Geometry check sheet. Reference: the model listing, model coordinates, mm. A direction names the side the tool comes from. Give positions to 0.01 mm unless a question says otherwise; leave off trailing zeros. Write each loop counter-clockwise with the first axis right and the second up, starting at its lowest first coordinate (ties: lowest second). Pieces come first, ordered by that corner, then holes. Notation, with made-up numbers: M 26,-35.5 L 71,-35.5 A26 cw 71,-21.5 Z; hole C 71.25,86 d11. An arc over 180 degrees is marked long. One line per item, written item: value. Start each with the question number.
1. Gauge pin test, flat ends, axial feed: pin 1 (3 mm diameter, centred on x = 10, z = 57, fed in from +Y); pin 2 (12 mm diameter, centred on y = -15.5, z = 158, fed in from +X); pin 3 (4 mm diameter, centred on x = -2.5, z = -13, fed in from +Y). Record the tip position at first contact, or that the pin passes through.
2. Cross-section at A-A on z = -31.7. Record the cut outline in (x, y), then the cut area to 3 significant figures.
3. Tool access check on faces 5 (the face through (-11, 17, 0)), 6 (the face through (-14.985, 0.66, 165.891)), 7 (the face through (8.06, -12.65, -29.52)), 8 (the face through (12, 0, -17.7)). Record the directions out of +Z, -Z, +X, -X, +Y, -Y that give a thin tool (end or side, any length) a straight path to the whole face; none if there is none.
4. Release check for a two-part mould opening along Z. For faces 1 (the face through (6, -6, 173.3)), 2 (the face through (-12, 0, -17.7)), 3 (the face through (-10, 0, -25)), 4 (the face through (-11, 17, 142.6)) record: pulls with the +Z half, pulls with the -Z half, needs draft (parallel to the pull), parting line crosses it, or undercut.
5. Cross-section at B-B on x = 17. Record the cut outline in (y, z) (3 decimals).
6. Scan lines: line 1 (Y direction, x = 0, z = 107); line 2 (Z direction, x = -7, y = -0.5); line 3 (Z direction, x = -7.5, y = -18). Record each from-to range of solid material in increasing order.
7. Cross-section at C-C on z = 60.5. Record the cut outline in (x, y), then the cut area to 3 significant figures.
from build123d import *

# Parameters (mm, degrees)
ESQUISSE1_R             = 20
BOSS_EXTRU_1_DEPTH      = 142.6
ESQUISSE2_R             = 20.8
BOSS_EXTRU_2_DEPTH      = 16.7
BOSS_EXTRU_5_START      = -159.3
ESQUISSE2_3_R           = 20.8
BOSS_EXTRU_5_DEPTH      = 16.7
ESQUISSE3_R             = 15
BOSS_EXTRU_6_DEPTH      = 27
ESQUISSE4_W             = 6
ESQUISSE4_H             = 30
ENL_V_MAT_EXTRU_1_DEPTH = 26
ESQUISSE5_R             = 6
ENL_V_MAT_EXTRU_2_DEPTH = 164.578024196
CHANFREIN1_SIZE         = 1
BOSS_EXTRU_7_START      = 14
ESQUISSE6_R             = 15
BOSS_EXTRU_7_DEPTH      = 14
ESQUISSE7_R             = 8
BOSS_EXTRU_8_DEPTH      = 8
CHANFREIN3_SIZE         = 1
ESQUISSE9_R             = 6.25
ENL_V_MAT_EXTRU_3_DEPTH = 100


with BuildPart() as part:
    # Esquisse1 → Boss.-Extru.1 (new body)
    with BuildSketch(Plane.XY):
        Circle(ESQUISSE1_R)
    extrude(amount=BOSS_EXTRU_1_DEPTH)

    # Esquisse2 → Boss.-Extru.2 (add)
    with BuildSketch(Plane.XY.offset(142.6)):
        Circle(ESQUISSE2_R)
    extrude(amount=BOSS_EXTRU_2_DEPTH)

    # Esquisse2_3 → Boss.-Extru.5 (add)
    with BuildSketch(Plane.XY.offset(142.6).offset(BOSS_EXTRU_5_START)):
        Circle(ESQUISSE2_3_R)
    extrude(amount=BOSS_EXTRU_5_DEPTH)

    # Esquisse3 → Boss.-Extru.6 (add)
    with BuildSketch(Plane(origin=(0, 0, -16.7), x_dir=(-1, 0, 0), z_dir=(0, 0, -1))):
        with Locations(Location((0, 0, 0), (0, 0, 180))):
            Circle(ESQUISSE3_R)
    extrude(amount=BOSS_EXTRU_6_DEPTH)

    # Esquisse4 → Enl_v. mat.-Extru.1 (cut)
    with BuildSketch(Plane(origin=(0, 0, -43.7), x_dir=(-1, 0, 0), z_dir=(0, 0, -1))):
        with Locations((-13, 0)):
            Rectangle(ESQUISSE4_W, ESQUISSE4_H)
        with Locations((13, 0)):
            Rectangle(ESQUISSE4_W, ESQUISSE4_H)
    extrude(amount=-ENL_V_MAT_EXTRU_1_DEPTH, mode=Mode.SUBTRACT)

    # Esquisse5 → Enl_v. mat.-Extru.2 (cut, through all)
    with BuildSketch(Plane(origin=(10, 0, 0), x_dir=(0, 0, -1), z_dir=(1, 0, 0))):
        with Locations((31.7, 0)):
            Circle(ESQUISSE5_R)
    extrude(amount=-ENL_V_MAT_EXTRU_2_DEPTH, mode=Mode.SUBTRACT)

    # Chanfrein1
    chanfrein1_edges = [part.edges().sort_by_distance(p)[0] for p in [
        (0, -15, -43.7),
        (0, 15, -43.7),
    ]]
    chamfer(chanfrein1_edges, length=CHANFREIN1_SIZE)

    # Esquisse6 → Boss.-Extru.7 (add)
    with BuildSketch(Plane.XY.offset(159.3).offset(BOSS_EXTRU_7_START)):
        Circle(ESQUISSE6_R)
    extrude(amount=-BOSS_EXTRU_7_DEPTH)

    # Esquisse7 → Boss.-Extru.8 (add)
    with BuildSketch(Plane.XY.offset(173.3)):
        Circle(ESQUISSE7_R)
    extrude(amount=BOSS_EXTRU_8_DEPTH)

    # Chanfrein3
    chanfrein3_edges = [part.edges().sort_by_distance(p)[0] for p in [
        (-15, 0, 173.3),
        (-8, 0, 181.3),
    ]]
    chamfer(chanfrein3_edges, length=CHANFREIN3_SIZE)

    # Esquisse9 → Enl_v. mat.-Extru.3 (cut)
    with BuildSketch(Plane.XY.offset(181.3)):
        Circle(ESQUISSE9_R)
    extrude(amount=-ENL_V_MAT_EXTRU_3_DEPTH, mode=Mode.SUBTRACT)


solid = part.part
Report:
1. pin 1: stops at y = 18.1
1. pin 2: stops at x = 18.5
1. pin 3: stops at y = 20.79
2. outline: M -10,-11.18 A15 ccw 10,-11.18 L 10,-6 L -10,-6 Z; M -10,6 L 10,6 L 10,11.18 A15 ccw -10,11.18 Z
2. area: 312 mm^2
3. face 5: none
3. face 6: +Z
3. face 7: -Z
3. face 8: -Z, +X, +Y, -Y
4. face 1: pulls with the +Z half
4. face 2: pulls with the -Z half
4. face 3: needs draft
4. face 4: undercut
5. outline: M -11.985,-16.7 L 11.985,-16.7 L 11.985,0 L 10.536,0 L 10.536,142.6 L 11.985,142.6 L 11.985,159.3 L -11.985,159.3 L -11.985,142.6 L -10.536,142.6 L -10.536,0 L -11.985,0 Z
6. line 1: y = -20 to -6.25, 6.25 to 20
6. line 2: z = -43.7 to -37.68, -25.72 to 181.28
6. line 3: z = -16.7 to 159.3
7. outline: C 0,0 d40
7. area: 1,260 mm^2
